from build123d import *

# Parameters (mm, degrees)
SKETCH_W  = 435
SKETCH_H  = 295
PAD_DEPTH = 14


with BuildPart() as part:
    # Sketch → Pad (new body)
    with BuildSketch(Plane.XY):
        Rectangle(SKETCH_W, SKETCH_H)
        Polygon((186.788842, -137.5), (-186.788842, -137.5), (-207.5, -116.788842), (-207.5, 116.788842), (-186.788842, 137.5), (186.788842, 137.5), (207.5, 116.788842), (207.5, -116.788842), align=None, mode=Mode.SUBTRACT)
    extrude(amount=PAD_DEPTH)


solid = part.part
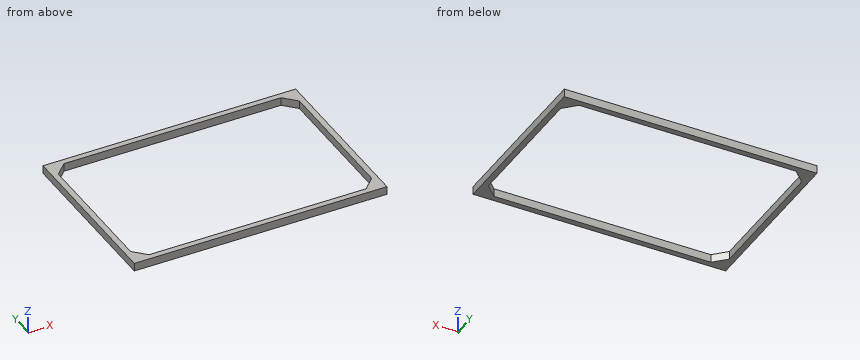
CAD build for the part. Positions are in the model's coordinates, mm. Give positions to 0.01 mm unless a question says otherwise; leave off trailing zeros. Write each loop counter-clockwise with the first axis right and the second up, starting at its lowest first coordinate (ties: lowest second). Pieces come first, ordered by that corner, then holes. Notation, with made-up numbers: M 8.25,-4.75 L 62.25,-4.75 A12 cw 62.25,13.25 Z; hole C 52.5,44 d1. An arc over 180 degrees is marked long. Put each result on its own line as item: value. Start each with the question number.
(1) Band-saw the part on B-B, the plane y = 32. Write the cut outline in (x, z).
(2) Band-saw the part on C-C, the plane z = 8. Write the cut outline in (x, y).
(3) Probe L1, parallel to Y at x = -51, z = 12.75; L2, parallel to X at y = -80.5, z = 13.25; L3, parallel to Y at x = 192.5, z = 3. List the from-to ranges inside material, lowest first.
(4) Band-saw the part on A-A, the plane x = -101. Write the cut outline in (y, z), and give its area (3 significant figures).
Response values:
1. outline: M -217.5,0 L -207.5,0 L -207.5,14 L -217.5,14 Z; M 207.5,0 L 217.5,0 L 217.5,14 L 207.5,14 Z
2. outline: M -217.5,-147.5 L 217.5,-147.5 L 217.5,147.5 L -217.5,147.5 Z; hole M -207.5,-116.79 L -186.79,-137.5 L 186.79,-137.5 L 207.5,-116.79 L 207.5,116.79 L 186.79,137.5 L -186.79,137.5 L -207.5,116.79 Z
3. L1: y = -147.5 to -137.5, 137.5 to 147.5
3. L2: x = -217.5 to -207.5, 207.5 to 217.5
3. L3: y = -147.5 to -131.79, 131.79 to 147.5
4. outline: M -147.5,0 L -137.5,0 L -137.5,14 L -147.5,14 Z; M 137.5,0 L 147.5,0 L 147.5,14 L 137.5,14 Z
4. area: 280 mm2
